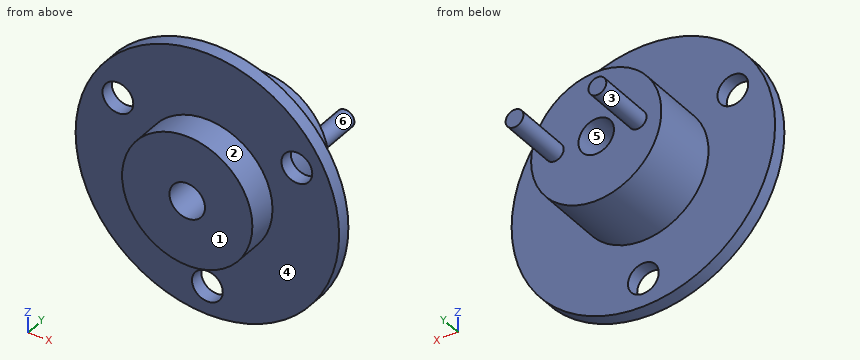
```python
from build123d import *

# Parameters (mm, degrees)
CROQUIS1_R              = 11
SALIENTE_EXTRUIR1_DEPTH = 19
CROQUIS2_R              = 22.25
SALIENTE_EXTRUIR2_DEPTH = 2.3
CROQUIS3_R              = 2.6
CORTAR_EXTRUIR1_DEPTH   = 2.3
CROQUIS4_R              = 3
CORTAR_EXTRUIR2_DEPTH   = 27.3
CROQUIS5_R              = 1.5
SALIENTE_EXTRUIR3_DEPTH = 10


with BuildPart() as part:
    # Croquis1 → Saliente-Extruir1 (new body)
    with BuildSketch(Plane(origin=(0, 0, 0), x_dir=(1, 0, 0), z_dir=(0, 1, 0))):
        Circle(CROQUIS1_R)
    extrude(amount=SALIENTE_EXTRUIR1_DEPTH)

    # Croquis2 → Saliente-Extruir2 (add)
    with BuildSketch(Plane(origin=(0, 5, 0), x_dir=(1, 0, 0), z_dir=(0, 1, 0))):
        Circle(CROQUIS2_R)
    extrude(amount=SALIENTE_EXTRUIR2_DEPTH)

    # Croquis3 → Cortar-Extruir1 (cut)
    with BuildSketch(Plane.XZ.offset(-5)):
        with Locations((15.112143296, 8.725)):
            Circle(CROQUIS3_R)
        with Locations((-15.112143296, 8.725)):
            Circle(CROQUIS3_R)
        with Locations((0, -17.45)):
            Circle(CROQUIS3_R)
    extrude(amount=-CORTAR_EXTRUIR1_DEPTH, mode=Mode.SUBTRACT)

    # Croquis4 → Cortar-Extruir2 (cut)
    with BuildSketch(Plane(origin=(0, 19, 0), x_dir=(1, 0, 0), z_dir=(0, 1, 0))):
        Circle(CROQUIS4_R)
    extrude(amount=-CORTAR_EXTRUIR2_DEPTH, mode=Mode.SUBTRACT)

    # Croquis5 → Saliente-Extruir3 (add)
    with BuildSketch(Plane(origin=(0, 19, 0), x_dir=(1, 0, 0), z_dir=(0, 1, 0))):
        with Locations((-7, 0)):
            Circle(CROQUIS5_R)
        with Locations((7, 0)):
            Circle(CROQUIS5_R)
    extrude(amount=SALIENTE_EXTRUIR3_DEPTH)


solid = part.part
```
Verification items for the finished model (mm, model axes). Face numbers are marked on the shaded views. A direction names the side the tool comes from. Coordinates: 2 decimals unless noted, no trailing zeros. Write each loop counter-clockwise with the first axis right and the second up, starting at its lowest first coordinate (ties: lowest second). Pieces come first, ordered by that corner, then holes. Notation, with made-up numbers: (49.25, 28.5) - (74.25, 28.5) arc R20 cw to (74.25, 65.5) - close; hole circle Ø2 at (-38.75, -6). An arc over 180 degrees is marked (long way). One line per question, with ' | ' between items. Start each with the question number.
1. Section check C-C (x = 0.5). Enter the section's corners in (y, z).
2. Section check D-D (z = -17.45). Enter the section's corners in (x, y).
3. Section check B-B (y = 22). Enter the section's corners in (x, z).
4. Draft check along Z on the marked faces 4, 5 and 6. Enter one of: released by +Z, released by -Z, zero draft, split by the parting line, or undercut.
5. Access from +Z, -Z, +X, -X, +Y, -Y to the whole of each face (thin tool, end or side, straight path). Record for the marked faces 1, 2 and 3.
6. Section check A-A (z = 0). Enter the section's corners in (x, y).
7. Material ranges on line 1 along Z through (x, y) = (0, 6.5); line 2 along Z through (x, y) = (0, 15); line 3 along Y through (x, z) = (11.5, -5), recorded low to high.
8. Gauge pin test, flat ends, axial feed: P1, Ø7, axis at x = -15.11, z = 8.72, coming from the -Y side; P2, Ø5, axis at x = 7, y = 12.5, coming from the -Z side; P3, Ø2, axis at x = -2.5, y = 6, coming from the +Z side. Record the tip position at first contact, or that the pin passes through.
Computed values:
1) outline: (0, -10.99) - (5, -10.99) - (5, -14.9) - (7.3, -14.9) - (7.3, -10.99) - (19, -10.99) - (19, -2.96) - (0, -2.96) - close; (0, 2.96) - (19, 2.96) - (19, 10.99) - (7.3, 10.99) - (7.3, 22.24) - (5, 22.24) - (5, 10.99) - (0, 10.99) - close; (5, -22.24) - (7.3, -22.24) - (7.3, -20) - (5, -20) - close
2) outline: (-13.8, 5) - (-2.6, 5) - (-2.6, 7.3) - (-13.8, 7.3) - close; (2.6, 5) - (13.8, 5) - (13.8, 7.3) - (2.6, 7.3) - close
3) outline: circle Ø3 at (-7, 0); circle Ø3 at (7, 0)
4) face 4: zero draft | face 5: undercut | face 6: split by the parting line
5) face 1: +Z, -Z, +X, -X, -Y | face 2: -Y | face 3: +Y
6) outline: (-22.25, 5) - (-11, 5) - (-11, 0) - (-3, 0) - (-3, 19) - (-5.5, 19) - (-5.5, 29) - (-8.5, 29) - (-8.5, 19) - (-11, 19) - (-11, 7.3) - (-22.25, 7.3) - close; (3, 0) - (11, 0) - (11, 5) - (22.25, 5) - (22.25, 7.3) - (11, 7.3) - (11, 19) - (8.5, 19) - (8.5, 29) - (5.5, 29) - (5.5, 19) - (3, 19) - close
7) line 1: -22.25 to -20.05, -14.85 to -3, 3 to 22.25 | line 2: -11 to -3, 3 to 11 | line 3: 5 to 7.3
8) P1: y = 5 | P2: z = -10.04 | P3: z = 22.2
